```python
from build123d import *

# Parameters (mm, degrees)
SKETCH_W        = 40
SKETCH_H        = 40
PAD_DEPTH       = 2
SKETCH001_W     = 33
SKETCH001_H     = 33
PAD001_DEPTH    = 6
SKETCH002_W     = 29
SKETCH002_H     = 29
POCKET_DEPTH    = 6
SKETCH003_W     = 10
SKETCH003_H     = 10
POCKET001_DEPTH = 15


with BuildPart() as part:
    # Sketch → Pad (new body)
    with BuildSketch(Plane.XY):
        Rectangle(SKETCH_W, SKETCH_H)
    extrude(amount=PAD_DEPTH)

    # Sketch001 (on Face6 of Pad) → Pad001 (join)
    with BuildSketch(Plane.XY.offset(2)):
        Rectangle(SKETCH001_W, SKETCH001_H)
    extrude(amount=PAD001_DEPTH)

    # Sketch002 (on Face11 of Pad001) → Pocket (cut)
    with BuildSketch(Plane.XY.offset(8)):
        Rectangle(SKETCH002_W, SKETCH002_H)
    extrude(amount=-POCKET_DEPTH, mode=Mode.SUBTRACT)

    # Sketch003 (on DatumPlane) → Pocket001 (cut)
    with BuildSketch(Plane.XZ.offset(20)):
        with Locations((0, 5.690688)):
            Rectangle(SKETCH003_W, SKETCH003_H)
    extrude(amount=-POCKET001_DEPTH, mode=Mode.SUBTRACT)


solid = part.part
```
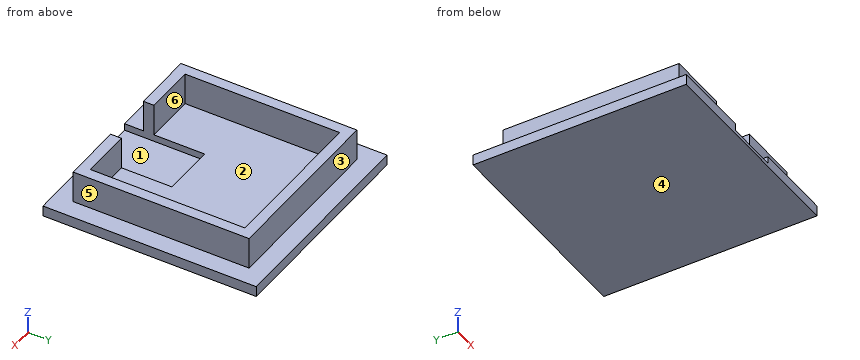
Part model, mm, in its own coordinate system. Face numbers are marked on the shaded views. A direction names the side the tool comes from. Round coordinates to 2 decimals unless told otherwise and drop trailing zeros. Write each loop counter-clockwise with the first axis right and the second up, starting at its lowest first coordinate (ties: lowest second). Pieces come first, ordered by that corner, then holes.
Item 1: Cut at A-A, the plane y = 14. Give the cut face in (x, z).
Results:
outline: (-20, 0) - (20, 0) - (20, 2) - (16.5, 2) - (16.5, 8) - (14.5, 8) - (14.5, 2) - (-14.5, 2) - (-14.5, 8) - (-16.5, 8) - (-16.5, 2) - (-20, 2) - close
Item 2: Drop flat-ended pins along their axis: pin 1 Ø1 at (y, z) = (-15, 5) entering from +X; pin 2 Ø20 at (x, y) = (-1.5, -4.5) entering from +Z; pin 3 Ø4 at (x, y) = (0, -8.5) entering from +Z. Give the stop position or say it passes through.
Results:
pin 1: stops at x = 16.5
pin 2: stops at z = 2
pin 3: stops at z = 0.69
Item 3: Two-plate mould, pull along Y, no slides. Class the marked faces 1, 2 and 3: +Y half, -Y half, draft (parallel to the pull), parting line (faces both ways), or undercut.
Results:
face 1: draft
face 2: undercut
face 3: +Y half
Item 4: Cut at C-C, the plane x = 1. Give the cut face in (y, z).
Results:
outline: (-20, 0) - (20, 0) - (20, 2) - (16.5, 2) - (16.5, 8) - (14.5, 8) - (14.5, 2) - (-5, 2) - (-5, 0.69) - (-20, 0.69) - close
Item 5: Which spindle directions (+Z, -Z, +X, -X, +Y, -Y) get a long thin tool onto all of the face, cutting with end or side? Do the marked faces 4, 5 and 6. Say none if no direction does.
Results:
face 4: -Z, +X, -X, +Y, -Y
face 5: +Z, +X, +Y, -Y
face 6: +Z
Item 6: Probe L1, parallel to X at y = -1.5, z = 5.75; L2, parallel to X at y = -15, z = 7.75. List the from-to ranges inside material, lowest first.
Results:
L1: x = -16.5 to -14.5, 14.5 to 16.5
L2: x = -16.5 to -5, 5 to 16.5
Item 7: Cut at B-B, the plane z = 1.25. Give the cut face in (x, y), plus the area to 3 significant figures.
Results:
outline: (-20, -20) - (-5, -20) - (-5, -5) - (5, -5) - (5, -20) - (20, -20) - (20, 20) - (-20, 20) - close
area: 1,450 mm2
